Verification items for the finished model (mm, model axes). Face numbers are marked on the shaded views. A direction names the side the tool comes from. Give positions to 0.01 mm unless a question says otherwise; leave off trailing zeros. Order: outer loops, then holes, each group sorted by start corner. A loop starts at its lowest first (then second) coordinate and runs counter-clockwise, first axis right, second up. Notation, with made-up numbers: (15, -0.75) - (58, -0.75) arc R15 ccw to (58, 4.25) - close; hole circle Ø11 at (-19.75, -30). An arc over 180 degrees is marked (long way). Answer as a JSON object with one key per item and string values.
```python
from build123d import *

# Parameters (mm, degrees)
F1_DEPTH = 25.4


with BuildPart() as f1:
    # F0 (on Front) → F1 (new body)
    with BuildSketch(Plane.XZ):
        with BuildLine():
            Line((101.6, 0), (0, 0))
            Line((0, 0), (0, -63.5))
            Line((0, -63.5), (6.35, -63.5))
            ThreePointArc((6.35, -63.5), (24.310512, -56.060512), (31.75, -38.1))
            ThreePointArc((31.75, -38.1), (35.469744, -29.119744), (44.45, -25.4))
            Line((44.45, -25.4), (76.2, -25.4))
            ThreePointArc((76.2, -25.4), (94.160512, -17.960512), (101.6, 0))
        make_face()
    extrude(amount=-F1_DEPTH)


solid = f1.part
```
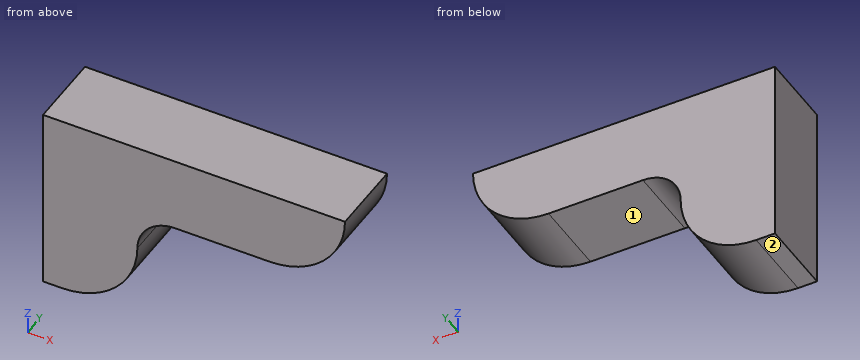
(1) Section check A-A (y = 21.25). Record the cut outline in (x, z), then the cut area to 3 significant figures.
Computed values:
{"outline": "(0, -63.5) - (6.35, -63.5) arc R25.4 ccw to (31.75, -38.1) arc R12.7 cw to (44.45, -25.4) - (76.2, -25.4) arc R25.4 ccw to (101.6, 0) - (0, 0) - close", "area": "3,550 mm²"}
(2) Access from +Z, -Z, +X, -X, +Y, -Y to the whole of each face (thin tool, end or side, straight path). Record for the marked faces 1 and 2.
Computed values:
{"face 1": "-Z, +X, +Y, -Y", "face 2": "-Z, +X, -X, +Y, -Y"}
(3) Material ranges on line 1 along Z through (x, y) = (55.5, 15); line 2 along Z through (x, y) = (6.5, 22.75); line 3 along X through (y, z) = (10, -51.5), recorded low to high. Write a range as [from, to].
Computed values:
{"line 1": "z = [-25.4, 0]", "line 2": "z = [-63.5, 0]", "line 3": "x = [0, 27.93]"}
(4) Section check B-B (x = 49). Record the cut outline in (y, z), then the cut area to 3 significant figures.
Computed values:
{"outline": "(0, -25.4) - (25.4, -25.4) - (25.4, 0) - (0, 0) - close", "area": "645 mm²"}
(5) Section check C-C (z = -10). Record the cut outline in (x, y), then the cut area to 3 significant figures.
Computed values:
{"outline": "(0, 0) - (99.55, 0) - (99.55, 25.4) - (0, 25.4) - close", "area": "2,530 mm²"}
(6) Gauge pin test, flat ends, axial feed: pin 1 Ø1.5 at (x, y) = (37, 5) entering from -Z; pin 2 Ø12 at (y, z) = (18, -38.5) entering from +X; pin 3 Ø8 at (x, y) = (42.5, 21) entering from -Z. Record the tip position at first contact, or that the pin passes through.
Computed values:
{"pin 1": "stops at z = -28.4", "pin 2": "stops at x = 33.05", "pin 3": "stops at z = -26.88"}
